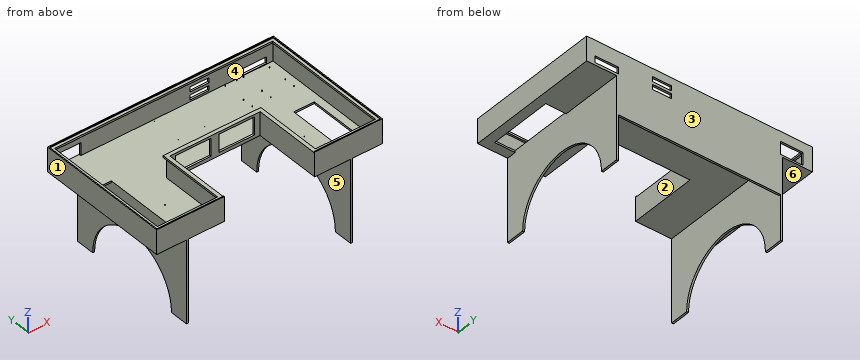
```python
from build123d import *

# Parameters (mm, degrees)
F1_DEPTH  = 12.7
F3_DEPTH  = 152.4
F4_R      = 1.9812
F5_DEPTH  = 6.35
F6_W      = 158.75
F6_H      = 44.45
F7_DEPTH  = 25.4
F8_W      = 127
F8_H      = 33.3375
F9_DEPTH  = 25.4
F10_R     = 1.5875
F11_DEPTH = 2.54
F12_W     = 138.649558
F12_H     = 568.248292
F12_H_2   = 428.248572
F13_DEPTH = 12.701
F14_R     = 3.175
F15_DEPTH = 3.175
F16_R     = 1.5875
F17_DEPTH = 3.175
F18_W     = 150.114
F18_H     = 86.106
F19_DEPTH = 25.4
F21_DEPTH = 6.35
F23_DEPTH = 12.7
F24_W     = 241.3
F24_H     = 120.65
F25_DEPTH = 25.4
F26_W     = 12.7
F26_H     = 914.4
F27_DEPTH = 558.8
F28_W     = 1094.300884
F28_H     = 12.7
F29_DEPTH = 254
F31_DEPTH = 1321.851442
F32_W     = 622.3
F32_H     = 457.2
F33_DEPTH = 25.4


with BuildPart() as f1:
    # F0 (on Top) → F1 (new body)
    with BuildSketch(Plane.XY):
        Polygon((0, 0), (0, 914.4), (-1524, 914.4), (-1524, 0), (-1066.8, 0), (-1066.8, 457.2), (-457.2, 457.2), (-457.2, 0), align=None)
    extrude(amount=F1_DEPTH)

    # F2 (on face) → F3 (join)
    with BuildSketch(Plane.XY.offset(12.7)):
        Polygon((-457.2, 0), (0, 0), (0, 914.4), (-1524, 914.4), (-1524, 0), (-1066.8, 0), (-1066.8, 457.2), (-457.2, 457.2), align=None)
        Polygon((-12.7, 901.7), (-12.7, 12.7), (-444.5, 12.7), (-444.5, 469.9), (-1079.5, 469.9), (-1079.5, 12.7), (-1511.3, 12.7), (-1511.3, 901.7), align=None, mode=Mode.SUBTRACT)
    extrude(amount=F3_DEPTH)

    # F4 (on face) → F5 (join)
    with BuildSketch(Plane.XY.offset(12.7)):
        with Locations((-345.44, 889.4318)):
            Circle(F4_R)
        with Locations((-266.7, 889.4318)):
            Circle(F4_R)
        with Locations((-220.98, 889.4318)):
            Circle(F4_R)
        with Locations((-63.5, 866.5718)):
            Circle(F4_R)
        with Locations((-63.5, 734.4918)):
            Circle(F4_R)
        with Locations((-220.98, 734.4918)):
            Circle(F4_R)
        with Locations((-345.44, 734.4918)):
            Circle(F4_R)
        with Locations((-345.44, 662.1018)):
            Circle(F4_R)
        with Locations((-220.98, 662.1018)):
            Circle(F4_R)
        with Locations((-63.5, 662.1018)):
            Circle(F4_R)
    extrude(amount=F5_DEPTH)

    # F6 (on face) → F7 (cut)
    with BuildSketch(Plane.XZ.offset(-901.7)):
        with Locations((-134.0866, 39.0398)):
            Rectangle(F6_W, F6_H)
    extrude(amount=-F7_DEPTH, mode=Mode.SUBTRACT)

    # F8 (on face) → F9 (cut)
    with BuildSketch(Plane.XZ.offset(-901.7)):
        with Locations((-508, 42.06875)):
            Rectangle(F8_W, F8_H)
        with Locations((-508, 94.45625)):
            Rectangle(F8_W, F8_H)
    extrude(amount=-F9_DEPTH, mode=Mode.SUBTRACT)

    # F10 (on face) → F11 (cut)
    with BuildSketch(Plane.XY.offset(12.7)):
        with Locations((-647.7, 889)):
            Circle(F10_R)
        with Locations((-647.7, 685.8)):
            Circle(F10_R)
        with Locations((-825.5, 889)):
            Circle(F10_R)
        with Locations((-825.5, 685.8)):
            Circle(F10_R)
    extrude(amount=-F11_DEPTH, mode=Mode.SUBTRACT)

    # F12 (on face) → F13 (cut, through all)
    with BuildSketch(Plane.XY.offset(12.7)):
        with Locations((-1391.175221, 347.624146)):
            Rectangle(F12_W, F12_H)
        with Locations((-132.824779, 277.624286)):
            Rectangle(F12_W, F12_H_2)
    extrude(amount=-F13_DEPTH, mode=Mode.SUBTRACT)

    # F14 (on face) → F15 (cut)
    with BuildSketch(Plane.XY.offset(12.7)):
        with Locations((-1231.9, 88.9)):
            Circle(F14_R)
        with Locations((-1231.9, 292.1)):
            Circle(F14_R)
        with Locations((-292.1, 292.1)):
            Circle(F14_R)
        with Locations((-292.1, 88.9)):
            Circle(F14_R)
    extrude(amount=-F15_DEPTH, mode=Mode.SUBTRACT)

    # F16 (on face) → F17 (cut)
    with BuildSketch(Plane.XY.offset(12.7)):
        with Locations((-1116.0125, 463.55)):
            Circle(F16_R)
        with Locations((-407.9875, 463.55)):
            Circle(F16_R)
    extrude(amount=-F17_DEPTH, mode=Mode.SUBTRACT)

    # F18 (on face) → F19 (cut)
    with BuildSketch(Plane.XZ.offset(-901.7)):
        with Locations((-1385.443, 55.753)):
            Rectangle(F18_W, F18_H)
    extrude(amount=-F19_DEPTH, mode=Mode.SUBTRACT)

    # F20 (on face) → F21 (cut)
    with BuildSketch(Plane.XY.offset(165.1)):
        Polygon((-1517.65, 908.05), (-1517.65, 6.35), (-1073.15, 6.35), (-1073.15, 463.55), (-450.85, 463.55), (-450.85, 6.35), (-6.35, 6.35), (-6.35, 908.05), align=None)
        Polygon((-1079.5, 12.7), (-1511.3, 12.7), (-1511.3, 901.7), (-12.7, 901.7), (-12.7, 12.7), (-444.5, 12.7), (-444.5, 469.9), (-1079.5, 469.9), align=None, mode=Mode.SUBTRACT)
    extrude(amount=-F21_DEPTH, mode=Mode.SUBTRACT)

    # F22 (on face) → F23 (join)
    with BuildSketch(Plane.XY.offset(158.75)):
        Polygon((-1511.3, 901.7), (-1511.3, 12.7), (-1079.5, 12.7), (-1079.5, 469.9), (-444.5, 469.9), (-444.5, 12.7), (-12.7, 12.7), (-12.7, 901.7), align=None)
        Polygon((-1092.2, 25.4), (-1498.6, 25.4), (-1498.6, 889), (-25.4, 889), (-25.4, 25.4), (-431.8, 25.4), (-431.8, 482.6), (-1092.2, 482.6), align=None, mode=Mode.SUBTRACT)
    extrude(amount=-F23_DEPTH)

    # F24 (on face) → F25 (cut)
    with BuildSketch(Plane.XZ.offset(-457.2)):
        with Locations((-908.05, 82.55)):
            Rectangle(F24_W, F24_H)
        with Locations((-615.95, 82.55)):
            Rectangle(F24_W, F24_H)
    extrude(amount=-F25_DEPTH, mode=Mode.SUBTRACT)

    # F26 (on face) → F27 (join)
    with BuildSketch(Plane(origin=(0, 0, 0), x_dir=(1, 0, 0), z_dir=(0, 0, -1))):
        with Locations((-1315.500442, -457.2)):
            Rectangle(F26_W, F26_H)
        with Locations((-208.499558, -457.2)):
            Rectangle(F26_W, F26_H)
    extrude(amount=F27_DEPTH)

    # F28 (on face) → F29 (join)
    with BuildSketch(Plane(origin=(0, 0, 0), x_dir=(1, 0, 0), z_dir=(0, 0, -1))):
        with Locations((-762, -908.05)):
            Rectangle(F28_W, F28_H)
    extrude(amount=F29_DEPTH)

    # F30 (on face) → F31 (cut, through all)
    with BuildSketch(Plane(origin=(-1321.850442, 0, 0), x_dir=(0, -1, 0), z_dir=(-1, 0, 0))):
        with BuildLine():
            Line((-787.4, -558.8), (-127, -558.8))
            ThreePointArc((-127, -558.8), (-457.2, -228.6), (-787.4, -558.8))
        make_face()
    extrude(amount=-F31_DEPTH, mode=Mode.SUBTRACT)

    # F32 (on face) → F33 (cut)
    with BuildSketch(Plane.XY.offset(158.75)):
        with Locations((-762, 234.95)):
            Rectangle(F32_W, F32_H)
    extrude(amount=F33_DEPTH, mode=Mode.SUBTRACT)


solid = f1.part
```
Geometry: final body of the model. Coordinates: model frame, mm. Face numbers are marked on the shaded views. A direction names the side the tool comes from. Round coordinates to 2 decimals unless told otherwise and drop trailing zeros. Order: outer loops, then holes, each group sorted by start corner. A loop starts at its lowest first (then second) coordinate and runs counter-clockwise, first axis right, second up. Notation, with made-up numbers: (-34.75, 85.5) -> (15.25, 85.5) arc R16 ccw to (15.25, 112.5) -> close; hole circle Ø5 at (39.25, 89.5). An arc over 180 degrees is marked (long way). Use one line per item in the form item = value. Start each with the question number.
1. Line query: probe 1 along X at (y, z) = (162.5, 123.5); probe 2 along X at (y, z) = (685.8, 10.95); probe 3 along Y at (x, z) = (-292, 11). Output: solid intervals per line, ascending.
2. Draft query along X for the marked faces 1, 2 and 3. Return one class per face: pulls with the +X half, pulls with the -X half, needs draft (parallel to the pull), parting line crosses it, or undercut.
3. Cut plane D-D (x = -1172.5). Return the cut outline in (y, z).
4. Pin query (flat end, axial travel): pin 1 Ø4 at (x, y) = (-1231.9, 88.9) entering from +Z (3 decimals); pin 2 Ø2 at (x, y) = (-221, 889.5) entering from +Z; pin 3 Ø1 at (x, y) = (-330.5, 512) entering from +Z. Return the tip coordinate at first contact, or that it passes through.
5. Reachability of the marked faces 4, 5 and 6 from +Z, -Z, +X, -X, +Y, -Y: full face, straight path, thin tool, end or side. Return the list, or none.
6. Cut plane C-C (z = -346.5). Return the cut outline in (x, y).
7. Cut plane A-A (x = -895.5). Return the cut outline in (y, z) (3 decimals), then the cut area to 3 significant figures.
8. Cut plane B-B (x = -543.5). Count the separate pieces of the cut face and the enclosed holes in it, then the cut area to 3 significant figures.
Solution:
q1.probe_1 = -1524 to -1511.3, -1079.5 to -1066.8, -457.2 to -444.5, -12.7 to 0
q1.probe_2 = -1524 to -827.09, -823.91 to -649.29, -646.11 to 0
q1.probe_3 = 0 to 85.73, 92.07 to 288.93, 295.27 to 914.4
q2.face_1 = pulls with the -X half
q2.face_2 = undercut
q2.face_3 = needs draft
q3.outline = (0, 0) -> (901.7, 0) -> (901.7, -254) -> (914.4, -254) -> (914.4, 165.1) -> (908.05, 165.1) -> (908.05, 158.75) -> (889, 158.75) -> (889, 146.05) -> (901.7, 146.05) -> (901.7, 12.7) -> (12.7, 12.7) -> (12.7, 146.05) -> (25.4, 146.05) -> (25.4, 158.75) -> (6.35, 158.75) -> (6.35, 165.1) -> (0, 165.1) -> close
q4.pin_1 = 9.525
q4.pin_2 = 158.75
q4.pin_3 = 12.7
q5.face_4 = none
q5.face_5 = -Z, -Y
q5.face_6 = -Z, -X, +Y, -Y
q6.outline = (-1321.85, 0) -> (-1309.15, 0) -> (-1309.15, 204.3) -> (-1321.85, 204.3) -> close; (-1321.85, 710.1) -> (-1309.15, 710.1) -> (-1309.15, 914.4) -> (-1321.85, 914.4) -> close; (-214.85, 0) -> (-202.15, 0) -> (-202.15, 204.3) -> (-214.85, 204.3) -> close; (-214.85, 710.1) -> (-202.15, 710.1) -> (-202.15, 914.4) -> (-214.85, 914.4) -> close
q7.outline = (457.2, 0) -> (901.7, 0) -> (901.7, -254) -> (914.4, -254) -> (914.4, 165.1) -> (908.05, 165.1) -> (908.05, 158.75) -> (889, 158.75) -> (889, 146.05) -> (901.7, 146.05) -> (901.7, 12.7) -> (469.9, 12.7) -> (469.9, 22.225) -> (457.2, 22.225) -> close; (457.2, 142.875) -> (469.9, 142.875) -> (469.9, 146.05) -> (482.6, 146.05) -> (482.6, 158.75) -> (457.2, 158.75) -> close
q7.area = 11,600 mm^2
q8.separate_pieces = 4
q8.enclosed_holes = 0
q8.area = 10,700 mm^2
